Check sheet for the modelled part. Datum: model origin and axes. Units: mm. A direction names the side the tool comes from. Coordinates: 2 decimals unless noted, no trailing zeros. Loops run counter-clockwise (first coordinate to the right, second up) from the corner with the lowest first, then second, coordinate; pieces in that order, holes last. Notation, with made-up numbers: (83, 45.25) -> (104, 45.25) arc R9 ccw to (104, 49.25) -> close; hole circle Ø9 at (-3, -1.5). An arc over 180 degrees is marked (long way). Use one line per item in the form item = value.
from build123d import *

# Parameters (mm, degrees)
BOX006_W        = 86
BOX006_H        = 42.2
BOX006_DEPTH    = 12
BOX007_W        = 82
BOX007_H        = 38.2
BOX007_DEPTH    = 10
SKETCH020_R     = 2.7
PAD016_DEPTH    = 14
SKETCH021_R     = 1.5
POCKET003_DEPTH = 14
BOX008_W        = 2
BOX008_H        = 15
BOX008_DEPTH    = 5
BOX009_W        = 27
BOX009_H        = 2
BOX009_DEPTH    = 1.5


with BuildPart() as part:
    # Box006 → Box006 (join)
    with BuildSketch(Plane.XY):
        with Locations((43, 21.1)):
            Rectangle(BOX006_W, BOX006_H)
    extrude(amount=BOX006_DEPTH)

    # Box007 → Box007 (cut)
    with BuildSketch(Plane(origin=(2, 2, 2), x_dir=(1, 0, 0), z_dir=(0, 0, 1))):
        with Locations((41, 19.1)):
            Rectangle(BOX007_W, BOX007_H)
    extrude(amount=BOX007_DEPTH, mode=Mode.SUBTRACT)

    # Sketch020 → Pad016 (join)
    with BuildSketch(Plane.XY):
        with Locations((5.25, 36.35)):
            Circle(SKETCH020_R)
        with Locations((80.75, 36.35)):
            Circle(SKETCH020_R)
        with Locations((80.75, 5.85)):
            Circle(SKETCH020_R)
        with Locations((5.25, 5.85)):
            Circle(SKETCH020_R)
    extrude(amount=PAD016_DEPTH)

    # Sketch021 → Pocket003 (cut)
    with BuildSketch(Plane.XY.offset(2)):
        with Locations((5.25, 36.35)):
            Circle(SKETCH021_R)
        with Locations((80.75, 36.35)):
            Circle(SKETCH021_R)
        with Locations((80.75, 5.85)):
            Circle(SKETCH021_R)
        with Locations((5.25, 5.85)):
            Circle(SKETCH021_R)
    extrude(amount=POCKET003_DEPTH, mode=Mode.SUBTRACT)

    # Box008 → Box008 (cut)
    with BuildSketch(Plane(origin=(0, 20, 4), x_dir=(1, 0, 0), z_dir=(0, 0, 1))):
        with Locations((1, 7.5)):
            Rectangle(BOX008_W, BOX008_H)
    extrude(amount=BOX008_DEPTH, mode=Mode.SUBTRACT)

    # Box009 → Box009 (cut)
    with BuildSketch(Plane(origin=(29.5, 0, 2), x_dir=(1, 0, 0), z_dir=(0, 0, 1))):
        with Locations((13.5, 1)):
            Rectangle(BOX009_W, BOX009_H)
    extrude(amount=BOX009_DEPTH, mode=Mode.SUBTRACT)


solid = part.part
(1) Mould release check, pull along Y, two halves, no side actions. Record for faces 6 (the flat face through (43, 1, 3.5)), 7 (the flat face through (42, 42.2, 6)), 8 (the cylindrical face through (82.18, 6.3, 7.92)): +Y half, -Y half, draft (parallel to the pull), parting line (faces both ways), or undercut.
Established:
face_6 = draft
face_7 = +Y half
face_8 = undercut
(2) Scan lines: line 1 along X through (y, z) = (5.85, 11.5); line 2 along Y through (x, z) = (80.75, 10.5); line 3 along Y through (x, z) = (42.5, 5.25). Record each from-to range of solid material in increasing order.
Established:
line_1 = 0 to 2, 2.55 to 3.75, 6.75 to 7.95, 78.05 to 79.25, 82.25 to 83.45, 84 to 86
line_2 = 0 to 2, 3.15 to 4.35, 7.35 to 8.55, 33.65 to 34.85, 37.85 to 39.05, 40.2 to 42.2
line_3 = 0 to 2, 40.2 to 42.2
(3) Section check B-B, the plane x = 36. Record the boundary of the cut face in (y, z), plus the area to 3 significant figures.
Established:
outline = (0, 0) -> (42.2, 0) -> (42.2, 12) -> (40.2, 12) -> (40.2, 2) -> (0, 2) -> close; (0, 3.5) -> (2, 3.5) -> (2, 12) -> (0, 12) -> close
area = 121 mm²
(4) Section check C-C, the plane x = 80.75. Record the boundary of the cut face in (y, z), plus the area to 3 significant figures.
Established:
outline = (0, 0) -> (42.2, 0) -> (42.2, 12) -> (40.2, 12) -> (40.2, 2) -> (39.05, 2) -> (39.05, 14) -> (37.85, 14) -> (37.85, 2) -> (34.85, 2) -> (34.85, 14) -> (33.65, 14) -> (33.65, 2) -> (8.55, 2) -> (8.55, 14) -> (7.35, 14) -> (7.35, 2) -> (4.35, 2) -> (4.35, 14) -> (3.15, 14) -> (3.15, 2) -> (2, 2) -> (2, 12) -> (0, 12) -> close
area = 182 mm²
(5) Section check D-D, the plane y = 36.35. Record the boundary of the cut face in (x, z).
Established:
outline = (0, 0) -> (86, 0) -> (86, 12) -> (84, 12) -> (84, 2) -> (83.45, 2) -> (83.45, 14) -> (82.25, 14) -> (82.25, 2) -> (79.25, 2) -> (79.25, 14) -> (78.05, 14) -> (78.05, 2) -> (7.95, 2) -> (7.95, 14) -> (6.75, 14) -> (6.75, 2) -> (3.75, 2) -> (3.75, 14) -> (2.55, 14) -> (2.55, 2) -> (2, 2) -> (2, 12) -> (0, 12) -> close
(6) Go/stop test with flat-tipped pins: P1, Ø1.5, axis at x = 51.5, y = 30, coming from the +Z side; P2, Ø1.6, axis at x = 1.5, y = 27.5, coming from the +Z side. Record where each tip stops, or that it passes through.
Established:
P1 = 2
P2 = 12
(7) Section check A-A, the plane y = 30. Record the boundary of the cut face in (x, z).
Established:
outline = (0, 0) -> (86, 0) -> (86, 12) -> (84, 12) -> (84, 2) -> (2, 2) -> (2, 4) -> (0, 4) -> close; (0, 9) -> (2, 9) -> (2, 12) -> (0, 12) -> close
(8) Tool access check on faces 1 (the flat face through (56.5, 1, 3)), 2 (the flat face through (86, 21, 6)), 3 (the flat face through (42, 0, 6)), 4 (the flat face through (1, 28, 9)), 5 (the flat face through (81, 6, 2)). Record the directions out of +Z, -Z, +X, -X, +Y, -Y that give a thin tool (end or side, any length) a straight path to the whole face; none if there is none.
Established:
face_1 = -Y
face_2 = +Z, -Z, +X, +Y, -Y
face_3 = +Z, -Z, +X, -X, -Y
face_4 = -X
face_5 = +Z
